Design review of the part built by this model. Coordinates are the model's own, in mm. Face numbers are marked on the shaded views. Coordinates: 2 decimals unless noted, no trailing zeros. Write each loop counter-clockwise with the first axis right and the second up, starting at its lowest first coordinate (ties: lowest second). Pieces come first, ordered by that corner, then holes.
Q1. The part is to be moulded in two halves that separate along Z. For the marked faces 1, 2, 3 and 4, say which applies: +Z half, -Z half, draft (parallel to the pull), parting line (faces both ways), or undercut.
Q2. Add section C-C, the plane y = -22. Give the boundary of the cut face in (x, z).
Q3. Add section B-B, the plane z = 0. Give the boundary of the cut face in (x, y).
Q4. Add section A-A, the plane y = 0. Give the boundary of the cut face in (x, z), plus the area to 3 significant figures.
Q5. Clearance check with flat-ended pins moving along their axes: pin 1 Ø12 at (y, z) = (40, -17) entering from -X; pin 2 Ø4 at (x, y) = (2.5, -4.5) entering from +Z; pin 3 Ø1 at (x, y) = (12, -23.5) entering from +Z; pin 4 Ø12.5 at (y, z) = (-54.35, 17.66) entering from -X. State where each tip first meets the part, or that it passes through.
Q6. To check wall thickness, follow probe 1 along Z at (x, y) = (17.5, 0); probe 2 along Y at (x, z) = (14.5, -43.5); probe 3 along Y at (x, z) = (18, 14). State the ranges of each line that lie inside material, in increasing order.
Q7. Add section D-D, the plane x = 13.25. Give the boundary of the cut face in (y, z).
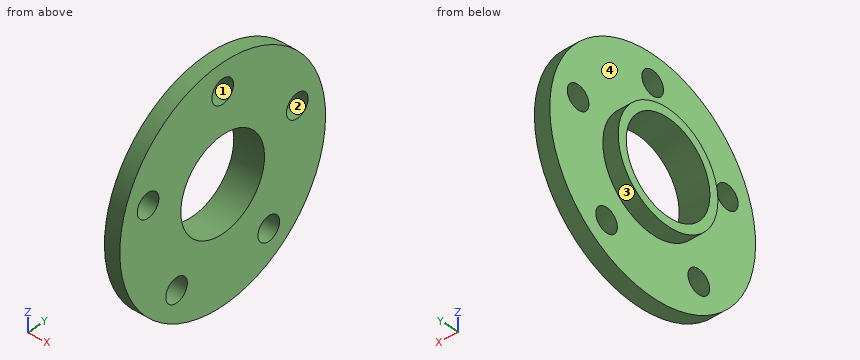
from build123d import *

# Parameters (mm, degrees)
F3_R            = 7.874
F4_DEPTH        = 10.161
F4_COPIES_COUNT = 5


# Not quite as in the source:
# - a pattern or mirror of a feature is missing from the dataset's text; its kind, count and spacing are read off the source's solid


with BuildPart() as f2:
    # F1 (on Front) → F2 (revolve)
    with BuildSketch(Plane.XZ):
        Polygon((0, 36.322), (0, 30.48), (20.32, 30.48), (20.32, 74.93), (10.16, 74.93), (10.16, 36.322), align=None)
    revolve(axis=Axis((6.4773708582, 0, 0), (1, 0, 0)))

    # F3 (on face) → F4 (cut, through all)
    with BuildSketch(Plane(origin=(10.16, 0, 0), x_dir=(0, -1, 0), z_dir=(-1, 0, 0))):
        with Locations((0, 57.15)):
            Circle(F3_R)
    f4 = extrude(amount=-F4_DEPTH, mode=Mode.SUBTRACT)

    # F4_copies: F4 ×5 about axis
    f4_copies_axis = Axis((0, 0, 0), (1, 0, 0))
    for i in range(1, F4_COPIES_COUNT):
        add(f4.rotate(f4_copies_axis, i * 360 / F4_COPIES_COUNT), mode=Mode.SUBTRACT)


solid = f2.part
Here are the results:
1. face 1: undercut
1. face 2: undercut
1. face 3: parting line
1. face 4: draft
2. outline: (0, -28.9) - (10.16, -28.9) - (10.16, -71.63) - (20.32, -71.63) - (20.32, -21.1) - (0, -21.1) - close; (0, 21.1) - (20.32, 21.1) - (20.32, 71.63) - (10.16, 71.63) - (10.16, 28.9) - (0, 28.9) - close
3. outline: (0, -36.32) - (10.16, -36.32) - (10.16, -74.93) - (20.32, -74.93) - (20.32, -30.48) - (0, -30.48) - close; (0, 30.48) - (20.32, 30.48) - (20.32, 74.93) - (10.16, 74.93) - (10.16, 36.32) - (0, 36.32) - close
4. outline: (0, -36.32) - (10.16, -36.32) - (10.16, -74.93) - (20.32, -74.93) - (20.32, -30.48) - (0, -30.48) - close; (0, 30.48) - (20.32, 30.48) - (20.32, 49.28) - (10.16, 49.28) - (10.16, 36.32) - (0, 36.32) - close; (10.16, 65.02) - (20.32, 65.02) - (20.32, 74.93) - (10.16, 74.93) - close
4. area: 862 mm2
5. pin 1: stops at x = 10.16
5. pin 2: stops at z = 36.24
5. pin 3: stops at z = 71.31
5. pin 4: passes through
6. probe 1: z = -74.93 to -30.48, 30.48 to 49.28, 65.02 to 74.93
6. probe 2: y = -61.01 to -40.98, -26.21 to 26.21, 40.98 to 61.01
6. probe 3: y = -73.61 to -61.32, -47.38 to -27.07, 27.07 to 47.38, 61.32 to 73.61
7. outline: circle Ø149.86 at (0, 0); hole circle Ø15.75 at (-54.35, 17.66); hole circle Ø15.75 at (-33.59, -46.24); hole circle Ø60.96 at (0, 0); hole circle Ø15.75 at (0, 57.15); hole circle Ø15.75 at (33.59, -46.24); hole circle Ø15.75 at (54.35, 17.66)
